Here's how the part is built. I have some questions about the finished solid (model axes, mm). Face numbers are marked on the shaded views. A direction names the side the tool comes from. Round coordinates to 2 decimals unless told otherwise and drop trailing zeros. Order: outer loops, then holes, each group sorted by start corner. A loop starts at its lowest first (then second) coordinate and runs counter-clockwise, first axis right, second up. Notation, with made-up numbers: (38, 82.25) - (68, 82.25) arc R21 ccw to (68, 96.25) - close; hole circle Ø9 at (67.25, 26.25). An arc over 180 degrees is marked (long way). One line per item, written item: value.
from build123d import *

# Parameters (mm, degrees)
SKETCH1_W            = 50.8
SKETCH1_H            = 43.815
SKETCH1_W_2          = 15.875
SKETCH1_H_2          = 7.62
SKETCH1_W_3          = 35.56
SKETCH1_H_3          = 5.08
BOSS_EXTRUDE1_DEPTH  = 3.175
SKETCH2_W            = 50.8
SKETCH2_H            = 43.815
SKETCH2_W_2          = 44.45
SKETCH2_H_2          = 37.465
BOSS_EXTRUDE2_DEPTH  = 8.255
SKETCH3_W            = 41.91
SKETCH3_H            = 2.54
BOSS_EXTRUDE3_DEPTH  = 11.43
SKETCH4_W            = 35.56
SKETCH4_H            = 2.54
CUT_EXTRUDE1_DEPTH   = 8.255
BOSS_EXTRUDE4_DEPTH  = 3.175
MIRROR2_COPY_1_DEPTH = 3.175
SKETCH7_W            = 15.875
SKETCH7_H            = 7.62
BOSS_EXTRUDE5_DEPTH  = 8.255
CUT_EXTRUDE2_START   = -11.43
CUT_EXTRUDE2_DEPTH   = 8.255
BOSS_EXTRUDE6_DEPTH  = 3.175
BOSS_EXTRUDE7_DEPTH  = 46.040436
SKETCH12_R           = 5.08
CUT_EXTRUDE3_DEPTH   = 54.813285309
SKETCH13_R           = 5.08
CUT_EXTRUDE4_DEPTH   = 71.721858561


with BuildPart() as part:
    # Sketch1 → Boss-Extrude1 (new body)
    with BuildSketch(Plane(origin=(0, 0, 0), x_dir=(1, 0, 0), z_dir=(0, 1, 0))):
        Rectangle(SKETCH1_W, SKETCH1_H)
        Rectangle(SKETCH1_W_2, SKETCH1_H_2, mode=Mode.SUBTRACT)
        with Locations((0, -11.1125)):
            Rectangle(SKETCH1_W_3, SKETCH1_H_3, mode=Mode.SUBTRACT)
    extrude(amount=BOSS_EXTRUDE1_DEPTH)

    # Sketch2 → Boss-Extrude2 (add)
    with BuildSketch(Plane(origin=(0, 3.175, 0), x_dir=(1, 0, 0), z_dir=(0, 1, 0))):
        Rectangle(SKETCH2_W, SKETCH2_H)
        Rectangle(SKETCH2_W_2, SKETCH2_H_2, mode=Mode.SUBTRACT)
    extrude(amount=BOSS_EXTRUDE2_DEPTH)

    # Sketch3 → Boss-Extrude3 (add)
    with BuildSketch(Plane(origin=(0, 11.43, 0), x_dir=(1, 0, 0), z_dir=(0, 1, 0))):
        with Locations((0, -23.1775)):
            Rectangle(SKETCH3_W, SKETCH3_H)
    extrude(amount=-BOSS_EXTRUDE3_DEPTH)

    # Sketch4 → Cut-Extrude1 (cut)
    with BuildSketch(Plane(origin=(0, 11.43, 0), x_dir=(1, 0, 0), z_dir=(0, 1, 0))):
        with Locations((0, -20.0025)):
            Rectangle(SKETCH4_W, SKETCH4_H)
    extrude(amount=-CUT_EXTRUDE1_DEPTH, mode=Mode.SUBTRACT)

    # Sketch5 → Boss-Extrude4 (add)
    with BuildSketch(Plane(origin=(0, 11.43, 0), x_dir=(1, 0, 0), z_dir=(0, 1, 0))):
        Polygon((-25.4, -16.51), (-30.48, -16.51), (-30.48, -5.08), (-25.4, -5.08), (-25.4, -8.255), (-27.305, -8.255), (-27.305, -13.335), (-25.4, -13.335), align=None)
    boss_extrude4 = extrude(amount=-BOSS_EXTRUDE4_DEPTH)

    # Mirror1: Boss-Extrude4 across plane
    add(boss_extrude4.mirror(Plane.XY))

    # Mirror2: Boss-Extrude4 across plane
    add(boss_extrude4.mirror(Plane(origin=(0, 0, 0), x_dir=(0, 0, 1), z_dir=(1, 0, 0))))

    # Mirror2 copy 1 sketch → Mirror2 copy 1 (add)
    with BuildSketch(Plane(origin=(0, 11.43, 0), x_dir=(-1, 0, 0), z_dir=(0, 1, 0))):
        Polygon((-25.4, -16.51), (-30.48, -16.51), (-30.48, -5.08), (-25.4, -5.08), (-25.4, -8.255), (-27.305, -8.255), (-27.305, -13.335), (-25.4, -13.335), align=None)
    extrude(amount=-MIRROR2_COPY_1_DEPTH)

    # Sketch7 → Boss-Extrude5 (add)
    with BuildSketch(Plane(origin=(0, 3.175, 0), x_dir=(1, 0, 0), z_dir=(0, 1, 0))):
        Polygon((-22.225, -18.7325), (-17.78, -18.7325), (-17.78, -8.5725), (17.78, -8.5725), (17.78, -18.7325), (22.225, -18.7325), (22.225, 18.7325), (-22.225, 18.7325), align=None)
        Rectangle(SKETCH7_W, SKETCH7_H, mode=Mode.SUBTRACT)
    extrude(amount=BOSS_EXTRUDE5_DEPTH)

    # Sketch8 → Cut-Extrude2 (cut)
    with BuildSketch(Plane(origin=(0, 11.43, 0), x_dir=(1, 0, 0), z_dir=(0, 1, 0)).offset(CUT_EXTRUDE2_START)):
        Polygon((-25.4, 21.9075), (-25.4, -21.9075), (-20.955, -21.9075), (-20.955, -5.3975), (20.955, -5.3975), (20.955, -21.9075), (25.4, -21.9075), (25.4, 21.9075), align=None)
    extrude(amount=CUT_EXTRUDE2_DEPTH, mode=Mode.SUBTRACT)

    # Sketch10 → Boss-Extrude6 (add)
    with BuildSketch(Plane(origin=(0, 4.091059817, -23.201553164), x_dir=(-1, 0, 0), z_dir=(0, 0.173648178, -0.984807753))):
        Polygon((-25.4, 7.452155165), (-36.134503848, -15.568062626), (5.592301438, -35.025591481), (25.4, 7.452155165), align=None)
    extrude(amount=-BOSS_EXTRUDE6_DEPTH)

    # Sketch11 → Boss-Extrude7 (add)
    with BuildSketch(Plane(origin=(23.71774367, 10.891742818, 1.920508126), x_dir=(0.06669094, 0.03062604, -0.997303547), z_dir=(0.906307787, 0.416197741, 0.073386891))):
        Polygon((24.765441235, -25.795675729), (29.775724817, -57.147861593), (57.992692094, -52.638606369), (57.491663736, -49.503387783), (32.409915045, -53.511614648), (28.401688179, -28.429865957), (53.48343687, -24.421639092), (52.982408512, -21.286420505), align=None)
    extrude(amount=-BOSS_EXTRUDE7_DEPTH)

    # Sketch12 → Cut-Extrude3 (cut, through all)
    with BuildSketch(Plane(origin=(12.416760179, -26.223291592, -4.623873831), x_dir=(0.906307787, 0.416197741, 0.073386891), z_dir=(-0.422618262, 0.892538935, 0.157378696))):
        with Locations((-9.550583138, 36.25947452)):
            Circle(SKETCH12_R)
        with Locations((15.849416862, 36.25947452)):
            Circle(SKETCH12_R)
    extrude(amount=-CUT_EXTRUDE3_DEPTH, mode=Mode.SUBTRACT)

    # Sketch13 → Cut-Extrude4 (cut, through all)
    with BuildSketch(Plane(origin=(0, 11.43, 0), x_dir=(1, 0, 0), z_dir=(0, 1, 0))):
        Circle(SKETCH13_R)
    extrude(amount=-CUT_EXTRUDE4_DEPTH, mode=Mode.SUBTRACT)


solid = part.part
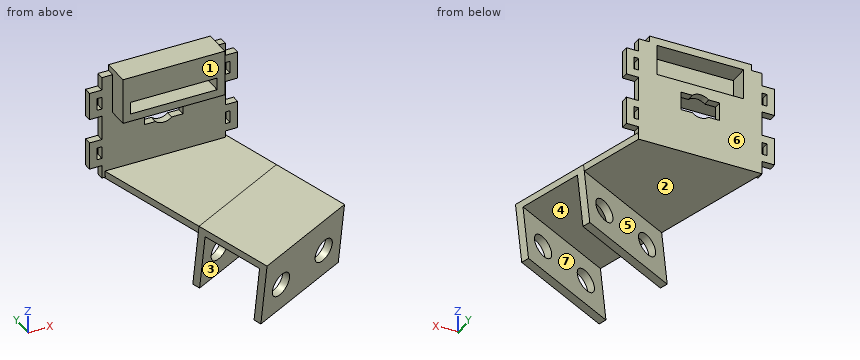
Q1. If we section it at C-C, the plane x = -13: Please give me the cut outline in (y, z) (1 decimal).
Results list:
outline: (-15.3, -23.4) - (-14.8, -26.5) - (11.4, -21.9) - (11.4, 8.6) - (0, 8.6) - (0, 5.4) - (8.3, 5.4) - (8.3, -19.2) - close; (0, 13.7) - (3.2, 13.7) - (3.2, 21.3) - (11.4, 21.3) - (11.4, 24.4) - (0, 24.4) - close
Q2. We'd pull the mould along Y, two halves only. Please class the marked faces 1, 2 and 3: released by +Y, released by -Y, zero draft, split by the parting line, or undercut.
Results list:
face 1: released by -Y
face 2: released by +Y
face 3: undercut
Q3. If we section it at D-D, the plane x = 1: Give the number of separate pieces and of enclosed holes in the cut face, then the cut area to 3 significant figures.
Results list:
separate pieces: 4
enclosed holes: 0
area: 389 mm²
Q4. If I drill on line 1 along Y through (x, z) = (-9.5, -10) (3 decimals); line 2 along Y through (x, z) = (20.5, 19.5); line 3 along Y through (x, z) = (21.5, -50), over which ranges is the centre line in solid material (lowest first)?
Results list:
line 1: 8.255 to 11.43
line 2: 0 to 11.43
line 3: -49.49 to -45.94, -17.48 to -13.92
Q5. Which directions (+Z, -Z, +X, -X, +Y, -Y) give clear straight access to the entire face, cutting with the end or side of a thin tool? Please do the marked faces 4, 5, 6 and 7.
Results list:
face 4: none
face 5: -X, +Y
face 6: +Z, -Z, +X, -X, +Y
face 7: -X
Q6. If we section it at A-A, the plane z = 10.5: Please give me the cut outline in (x, y) (3 decimals).
Results list:
outline: (-30.48, 8.255) - (-27.305, 8.255) - (-27.305, 11.43) - (-30.48, 11.43) - close; (-25.4, 8.255) - (-20.955, 8.255) - (-20.955, 0) - (-17.78, 0) - (-17.78, 11.43) - (-25.4, 11.43) - close; (17.78, 0) - (20.955, 0) - (20.955, 8.255) - (25.4, 8.255) - (25.4, 11.43) - (17.78, 11.43) - close; (27.305, 8.255) - (30.48, 8.255) - (30.48, 11.43) - (27.305, 11.43) - close
Q7. If we section it at B-B, the plane z = -0.5: Please give me the cut outline in (x, y) (1 decimal), then the cut area to 3 significant figures.
Results list:
outline: (-25.4, 8.3) - (-7.9, 8.3) - (-7.9, 11.4) - (-25.4, 11.4) - close; (7.9, 8.3) - (25.4, 8.3) - (25.4, 11.4) - (7.9, 11.4) - close
area: 111 mm²
Q8. Will these pins go through, and if not, where does the flat tip stop? pin 1 (1.6 mm diameter, centred on x = -27.5, y = 10, fed in from -Z); pin 2 (1 mm diameter, centred on x = -15.5, z = -7.5, fed in from -Y) (3 decimals); pin 3 (0.7 mm diameter, centred on x = -24.5, y = 9, fed in from -Z).
Results list:
pin 1: z = -16.51
pin 2: y = 8.255
pin 3: z = -22.36
